```python
from build123d import *

# Parameters (mm, degrees)
EXTRUDE_1_DEPTH     = 94
SKETCH_2_R          = 1.2
CUT_EXTRUDE_1_DEPTH = 95.382413616


with BuildPart() as part:
    # 草图1 → 凸台-拉伸1 (new body)
    with BuildSketch(Plane(origin=(0, 0, 0), x_dir=(1, 0, 0), z_dir=(0, 1, 0))):
        Polygon((0, 0), (0, 2.6), (1, 2.6), (1, 3.6), (0, 3.6), (0, 4.8), (7, 4.8), (7, 3.6), (6, 3.6), (6, 2.6), (7, 2.6), (7, 0), align=None)
    extrude(amount=EXTRUDE_1_DEPTH)

    # 草图2 → 切除-拉伸1 (cut, through all)
    with BuildSketch(Plane(origin=(0, 0, -4.8), x_dir=(-1, 0, 0), z_dir=(0, 0, -1))):
        with Locations((-3.5, 62)):
            Circle(SKETCH_2_R)
        with Locations((-3.5, 77)):
            Circle(SKETCH_2_R)
        with Locations((-3.5, 47)):
            Circle(SKETCH_2_R)
        with Locations((-3.5, 32)):
            Circle(SKETCH_2_R)
        with Locations((-3.5, 17)):
            Circle(SKETCH_2_R)
        with Locations((-3.5, 92)):
            Circle(SKETCH_2_R)
        with Locations((-3.5, 2)):
            Circle(SKETCH_2_R)
    extrude(amount=-CUT_EXTRUDE_1_DEPTH, mode=Mode.SUBTRACT)


solid = part.part
```
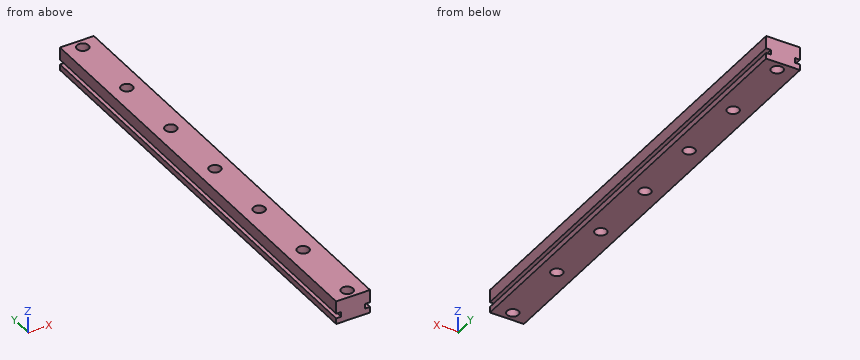
Verification items for the finished model (mm, model axes). Round coordinates to 2 decimals unless told otherwise and drop trailing zeros. Write each loop counter-clockwise with the first axis right and the second up, starting at its lowest first coordinate (ties: lowest second). Pieces come first, ordered by that corner, then holes.
1. Scan lines: L1, parallel to Z at x = 6.5, y = 24.5; L2, parallel to X at y = 34.5, z = -2.85. Record each from-to range of solid material in increasing order.
2. Section check C-C on y = 9. Enter the section's corners in (x, z).
3. Section check A-A on x = 3.5. State how many separate pieces and enclosed holes the cut face has, plus the area to 3 significant figures.
4. Gauge pin test, flat ends, axial feed: P1, Ø2, axis at x = 3.5, y = 17, coming from the +Z side; P2, Ø0.5, axis at y = 60, z = -3, coming from the +X side; P3, Ø0.5, axis at y = 67, z = -3, coming from the -X side. Record the tip position at first contact, or that the pin passes through.
5. Section check D-D on z = -1.4. Enter the section's corners in (x, y).
6. Section check B-B on y = 92. Enter the section's corners in (x, z), plus the area to 3 significant figures.
Answer:
1. L1: z = -4.8 to -3.6, -2.6 to 0
1. L2: x = 1 to 6
2. outline: (0, -4.8) - (7, -4.8) - (7, -3.6) - (6, -3.6) - (6, -2.6) - (7, -2.6) - (7, 0) - (0, 0) - (0, -2.6) - (1, -2.6) - (1, -3.6) - (0, -3.6) - close
3. separate pieces: 8
3. enclosed holes: 0
3. area: 371 mm2
4. P1: passes through
4. P2: stops at x = 6
4. P3: stops at x = 1
5. outline: (0, 0) - (7, 0) - (7, 94) - (0, 94) - close; hole circle Ø2.4 at (3.5, 2); hole circle Ø2.4 at (3.5, 17); hole circle Ø2.4 at (3.5, 32); hole circle Ø2.4 at (3.5, 47); hole circle Ø2.4 at (3.5, 62); hole circle Ø2.4 at (3.5, 77); hole circle Ø2.4 at (3.5, 92)
6. outline: (0, -4.8) - (2.3, -4.8) - (2.3, 0) - (0, 0) - (0, -2.6) - (1, -2.6) - (1, -3.6) - (0, -3.6) - close; (4.7, -4.8) - (7, -4.8) - (7, -3.6) - (6, -3.6) - (6, -2.6) - (7, -2.6) - (7, 0) - (4.7, 0) - close
6. area: 20.1 mm2
